```python
from build123d import *

# Parameters (mm, degrees)
SKETCH1_R           = 63.5
BOSS_EXTRUDE1_DEPTH = 101.6
SKETCH2_R           = 25.4
CUT_EXTRUDE1_DEPTH  = 88.9
FILLET1_SIZE        = 7.62


with BuildPart() as part:
    # Sketch1 → Boss-Extrude1 (new body)
    with BuildSketch(Plane(origin=(0, 0, 0), x_dir=(1, 0, 0), z_dir=(0, 1, 0))):
        with Locations(Location((0, 0, 0), (0, 0, 270))):
            Circle(SKETCH1_R)
    extrude(amount=BOSS_EXTRUDE1_DEPTH)

    # Sketch2 → Cut-Extrude1 (cut)
    with BuildSketch(Plane(origin=(0, 101.6, 0), x_dir=(1, 0, 0), z_dir=(0, 1, 0))):
        with Locations(Location((0, 0, 0), (0, 0, 270))):
            Circle(SKETCH2_R)
    extrude(amount=-CUT_EXTRUDE1_DEPTH, mode=Mode.SUBTRACT)

    # Fillet1
    fillet1_edges = [part.edges().sort_by_distance(p)[0] for p in [
        (0, 101.6, -63.5),
    ]]
    chamfer(fillet1_edges, length=FILLET1_SIZE)


solid = part.part
```
Check sheet for the modelled part. Datum: model origin and axes. Units: mm. A direction names the side the tool comes from. Give positions to 0.01 mm unless a question says otherwise; leave off trailing zeros. Write each loop counter-clockwise with the first axis right and the second up, starting at its lowest first coordinate (ties: lowest second). Pieces come first, ordered by that corner, then holes. Notation, with made-up numbers: (71.25, 8) - (126.25, 8) arc R13 ccw to (126.25, 16) - close; hole circle Ø10 at (52, 83). An arc over 180 degrees is marked (long way). Answer as a JSON object with one key per item and string values. Group by question number.
1) Access from +Z, -Z, +X, -X, +Y, -Y to the whole of each face (thin tool, end or side, straight path). Record for faces 1 (the face through (-15.456, 57.772, -20.157)), 2 (the face through (1, 0, -1)).
2) Thickness scan on probe 1 along X at (y, z) = (36.5, 0); probe 2 along Y at (x, z) = (-4, -1); probe 3 along Y at (x, z) = (53, -32.5). Record the ranges inside material, lowest first. Write a range as from..to.
3) Depth check by flat-ended pin: P1, Ø10, axis at x = -36, y = 52, coming from the +Z side; P2, Ø10, axis at x = -39.5, y = 46, coming from the -Z side; P3, Ø5, axis at x = 25.5, y = 42.5, coming from the -Z side. Enter the tip coordinate at first touch or a pass-through.
4) Release check for a two-part mould opening along X. For faces 3 (the face through (-12, 101.6, 24)), 4 (the face through (0, 12.7, 0)), 5 (the face through (-61.99, 46.33, -13.77)) record: pulls with the +X half, pulls with the -X half, needs draft (parallel to the pull), parting line crosses it, or undercut.
5) Sectioned sample at C-C (y = 56.5). Record the cut outline in (x, z).
6) Sectioned sample at B-B (x = 0). Record the cut outline in (y, z), then the cut area to 3 significant figures.
7) Sectioned sample at A-A (z = 0). Record the cut outline in (x, y), then the cut area to 3 significant figures.
Geometry results:
{
 "1": {"face 1": "+Y", "face 2": "+Z, -Z, +X, -X, -Y"},
 "2": {"probe 1": "x = -63.5..-25.4, 25.4..63.5", "probe 2": "y = 0..12.7", "probe 3": "y = 0..95.31"},
 "3": {"P1": "stops at z = 55.42", "P2": "stops at z = -53.31", "P3": "stops at z = -59.19"},
 "4": {"face 3": "needs draft", "face 4": "undercut", "face 5": "parting line crosses it"},
 "5": {"outline": "circle Ø127 at (0, 0); hole circle Ø50.8 at (0, 0)"},
 "6": {"outline": "(0, -63.5) - (93.98, -63.5) - (101.6, -55.88) - (101.6, -25.4) - (12.7, -25.4) - (12.7, 25.4) - (101.6, 25.4) - (101.6, 55.88) - (93.98, 63.5) - (0, 63.5) - close", "area": "8,330 mm^2"},
 "7": {"outline": "(-63.5, 0) - (63.5, 0) - (63.5, 93.98) - (55.88, 101.6) - (25.4, 101.6) - (25.4, 12.7) - (-25.4, 12.7) - (-25.4, 101.6) - (-55.88, 101.6) - (-63.5, 93.98) - close", "area": "8,330 mm^2"}
}
